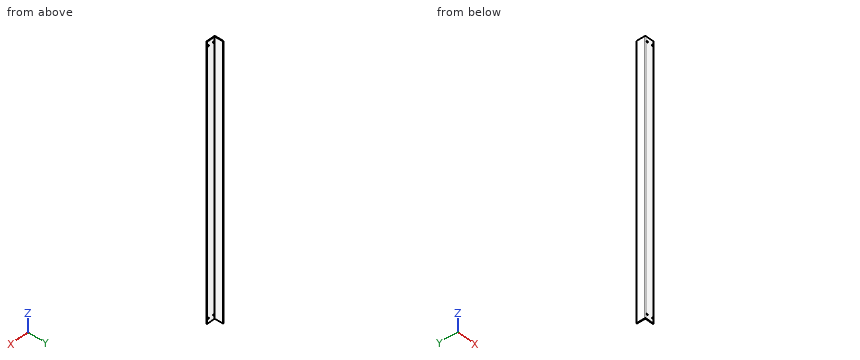
```python
from build123d import *

# Parameters (mm, degrees)
BOSS_EXTRUDE1_DEPTH = 1200
CUT_EXTRUDE1_REACH  = 1203.236
SKETCH2_R           = 3


with BuildPart() as part:
    # Sketch1 → Boss-Extrude1 (new body)
    with BuildSketch(Plane.XY):
        with BuildLine():
            Line((0, 3), (0, 40))
            Line((0, 40), (3, 40))
            Line((3, 40), (3, 3.5))
            ThreePointArc((3, 3.5), (3.146446609, 3.146446609), (3.5, 3))
            Line((3.5, 3), (40, 3))
            Line((40, 3), (40, 0))
            Line((40, 0), (3, 0))
            ThreePointArc((3, 0), (0.878679656, 0.878679656), (0, 3))
        make_face()
    extrude(amount=BOSS_EXTRUDE1_DEPTH)

    # Sketch2 → Cut-Extrude1 (cut, up to next)
    with BuildSketch(Plane(origin=(0, 3, 0), x_dir=(1, 0, 0), z_dir=(0, 1, 0)), mode=Mode.PRIVATE) as cut_extrude1_sk1:
        with Locations(Location((9, -1180, 0), (0, 0, 270))):
            Circle(SKETCH2_R)
    cut_extrude1_tool1 = extrude(cut_extrude1_sk1.sketch, amount=-CUT_EXTRUDE1_REACH, mode=Mode.PRIVATE) & part.part
    # Sketch2 → Cut-Extrude1 (cut, up to next)
    with BuildSketch(Plane(origin=(0, 3, 0), x_dir=(1, 0, 0), z_dir=(0, 1, 0)), mode=Mode.PRIVATE) as cut_extrude1_sk2:
        with Locations(Location((34, -1180, 0), (0, 0, 270))):
            Circle(SKETCH2_R)
    cut_extrude1_tool2 = extrude(cut_extrude1_sk2.sketch, amount=-CUT_EXTRUDE1_REACH, mode=Mode.PRIVATE) & part.part
    # Sketch2 → Cut-Extrude1 (cut, up to next)
    with BuildSketch(Plane(origin=(0, 3, 0), x_dir=(1, 0, 0), z_dir=(0, 1, 0)), mode=Mode.PRIVATE) as cut_extrude1_sk3:
        with Locations(Location((9, -20, 0), (0, 0, 270))):
            Circle(SKETCH2_R)
    cut_extrude1_tool3 = extrude(cut_extrude1_sk3.sketch, amount=-CUT_EXTRUDE1_REACH, mode=Mode.PRIVATE) & part.part
    # Sketch2 → Cut-Extrude1 (cut, up to next)
    with BuildSketch(Plane(origin=(0, 3, 0), x_dir=(1, 0, 0), z_dir=(0, 1, 0)), mode=Mode.PRIVATE) as cut_extrude1_sk4:
        with Locations(Location((34, -20, 0), (0, 0, 270))):
            Circle(SKETCH2_R)
    cut_extrude1_tool4 = extrude(cut_extrude1_sk4.sketch, amount=-CUT_EXTRUDE1_REACH, mode=Mode.PRIVATE) & part.part
    add(cut_extrude1_tool1.solids().sort_by_distance((9, 3, 1180))[0], mode=Mode.SUBTRACT)
    add(cut_extrude1_tool2.solids().sort_by_distance((34, 3, 1180))[0], mode=Mode.SUBTRACT)
    add(cut_extrude1_tool3.solids().sort_by_distance((9, 3, 20))[0], mode=Mode.SUBTRACT)
    add(cut_extrude1_tool4.solids().sort_by_distance((34, 3, 20))[0], mode=Mode.SUBTRACT)


solid = part.part
```
Geometry: final body of the model. Coordinates: model frame, mm. Coordinates: 2 decimals unless noted, no trailing zeros. Order: outer loops, then holes, each group sorted by start corner. A loop starts at its lowest first (then second) coordinate and runs counter-clockwise, first axis right, second up. Notation, with made-up numbers: (48, 69) -> (59, 69) arc R22 cw to (59, 104) -> close; hole circle Ø2 at (-38, 72). An arc over 180 degrees is marked (long way). Write each question's results on one line, items separated by ' | '. Start each with the question number.
1) Material intervals for line 1 along X through (y, z) = (2.35, 1180); line 2 along X through (y, z) = (2, 20); line 3 along Y through (x, z) = (30.5, 179), sorted ascending.
2) Cut plane A-A, the plane z = 183. Output: boundary loops of the cut face in (x, y).
3) First-contact query: pin 1 (9.5 mm diameter, centred on x = 9, z = 1180, fed in from +Y); pin 2 (1.5 mm diameter, centred on y = 10, z = 542.5, fed in from +X). Flat tips, straight axial feed; report the tip coordinate or a pass-through.
4) Cut plane B-B, the plane x = 18. Output: boundary loops of the cut face in (y, z), and give its area (3 significant figures).
Checks:
1) line 1: 0.07 to 6, 12 to 31, 37 to 40 | line 2: 0.17 to 6, 12 to 31, 37 to 40 | line 3: 0 to 3
2) outline: (0, 3) arc R3 ccw to (3, 0) -> (40, 0) -> (40, 3) -> (3.5, 3) arc R0.5 cw to (3, 3.5) -> (3, 40) -> (0, 40) -> close
3) pin 1: y = 3 | pin 2: x = 3
4) outline: (0, 0) -> (3, 0) -> (3, 1200) -> (0, 1200) -> close | area: 3,600 mm^2
